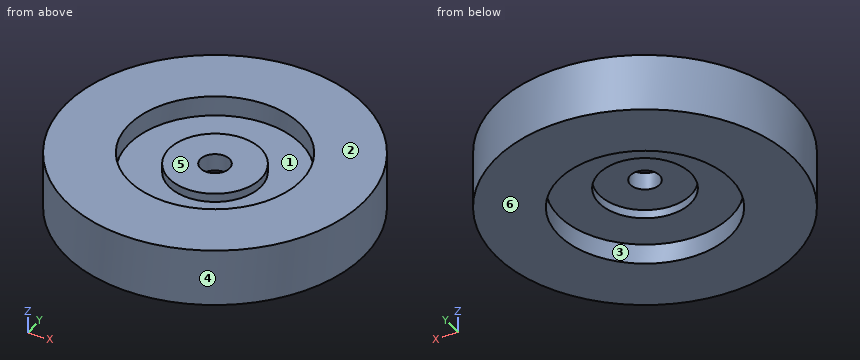
```python
from build123d import *

# Parameters (mm, degrees)
CROQUIS1_R              = 260
CROQUIS1_R_2            = 150
SALIENTE_EXTRUIR1_DEPTH = 50
CROQUIS1_3_R            = 150
CROQUIS1_3_R_2          = 80
SALIENTE_EXTRUIR2_DEPTH = 15
CROQUIS1_4_R            = 80
CROQUIS1_4_R_2          = 25.4
SALIENTE_EXTRUIR3_DEPTH = 30


with BuildPart() as part:
    # Croquis1 → Saliente-Extruir1 (new, symmetric)
    with BuildSketch(Plane.XY):
        Circle(CROQUIS1_R)
        Circle(CROQUIS1_R_2, mode=Mode.SUBTRACT)
    extrude(amount=SALIENTE_EXTRUIR1_DEPTH, both=True)

    # Croquis1<3> → Saliente-Extruir2 (add, symmetric)
    with BuildSketch(Plane.XY):
        Circle(CROQUIS1_3_R)
        Circle(CROQUIS1_3_R_2, mode=Mode.SUBTRACT)
    extrude(amount=SALIENTE_EXTRUIR2_DEPTH, both=True)

    # Croquis1<4> → Saliente-Extruir3 (add)
    with BuildSketch(Plane.XY):
        Circle(CROQUIS1_4_R)
        Circle(CROQUIS1_4_R_2, mode=Mode.SUBTRACT)
    extrude(amount=SALIENTE_EXTRUIR3_DEPTH)


solid = part.part
```
Geometry check sheet. Reference: the model listing, model coordinates, mm. Face numbers are marked on the shaded views. A direction names the side the tool comes from. Round coordinates to 2 decimals unless told otherwise and drop trailing zeros. Loops run counter-clockwise (first coordinate to the right, second up) from the corner with the lowest first, then second, coordinate; pieces in that order, holes last. Notation, with made-up numbers: M 43,69 L 79,69 A16 cw 79,77 Z; hole C 44,2 d8. An arc over 180 degrees is marked long. Return JSON: item names as keys, results as strings. Group by question number.
(1) Section check C-C, the plane z = -36.5. Enter the section's corners in (x, y), and give its area (3 significant figures).
(2) Scan lines: line 1 along Y through (x, z) = (0, -38); line 2 along Z through (x, y) = (48, 65.5); line 3 along Y through (x, z) = (0, -5). Record each from-to range of solid material in increasing order. Write a range as [from, to].
(3) Go/stop test with flat-tipped pins: pin 1 (10 mm diameter, centred on x = 123.5, y = -15.5, fed in from +Z); pin 2 (1 mm diameter, centred on y = 87, z = -4.5, fed in from -X); pin 3 (1.5 mm diameter, centred on x = -192, z = -34.5, fed in from +Y). Record where each tip stops, or that it passes through.
(4) Mould release check, pull along Y, two halves, no side actions. Record for the marked faces 4, 5 and 6: pulls with the +Y half, pulls with the -Y half, needs draft (parallel to the pull), parting line crosses it, or undercut.
(5) Set-up check for the marked faces 1, 2 and 3: record each of +Z, -Z, +X, -X, +Y, -Y from which the full face is reachable in a straight line by a thin tool's end or side.
(6) Section check A-A, the plane x = 0. Enter the section's corners in (y, z).
(7) Section check D-D, the plane x = -129. Enter the section's corners in (y, z).
Data:
{
 "1": {"outline": "C 0,0 d520; hole C 0,0 d300", "area": "142,000 mm²"},
 "2": {"line 1": "[-260, -150], [150, 260]", "line 2": "[-15, 15]", "line 3": "[-260, -80], [80, 260]"},
 "3": {"pin 1": "z = 15", "pin 2": "x = -245.19", "pin 3": "y = 176.13"},
 "4": {"face 4": "parting line crosses it", "face 5": "undercut", "face 6": "needs draft"},
 "5": {"face 1": "+Z", "face 2": "+Z, +X, -X, +Y, -Y", "face 3": "-Z"},
 "6": {"outline": "M -260,-50 L -150,-50 L -150,-15 L -80,-15 L -80,0 L -25.4,0 L -25.4,30 L -80,30 L -80,15 L -150,15 L -150,50 L -260,50 Z; M 25.4,0 L 80,0 L 80,-15 L 150,-15 L 150,-50 L 260,-50 L 260,50 L 150,50 L 150,15 L 80,15 L 80,30 L 25.4,30 Z"},
 "7": {"outline": "M -225.74,-50 L -76.54,-50 L -76.54,-15 L 76.54,-15 L 76.54,-50 L 225.74,-50 L 225.74,50 L 76.54,50 L 76.54,15 L -76.54,15 L -76.54,50 L -225.74,50 Z"}
}
